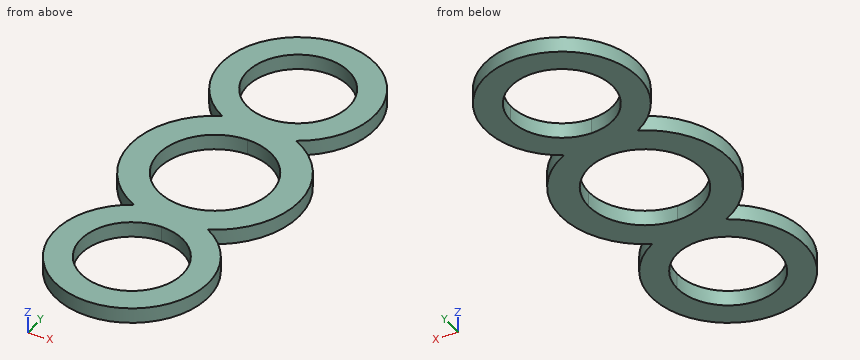
from build123d import *

# Parameters (mm, degrees)
F1_DEPTH = 3


with BuildPart() as f1:
    # F0 (on Top) → F1 (new body)
    with BuildSketch(Plane.XY):
        with BuildLine():
            ThreePointArc((7.205074, 14.84375), (0, 43), (-7.205074, 14.84375))
            ThreePointArc((-7.205074, 14.84375), (-16.5, 0), (-7.205074, -14.84375))
            ThreePointArc((-7.205074, -14.84375), (0, -43), (7.205074, -14.84375))
            ThreePointArc((7.205074, -14.84375), (16.5, 0), (7.205074, 14.84375))
        make_face()
        with BuildLine():
            ThreePointArc((9.95, -28), (-7.035712, -35.035712), (0, -18.05))
            ThreePointArc((0, -18.05), (7.035712, -20.964288), (9.95, -28))
        make_face(mode=Mode.SUBTRACT)
        with BuildLine():
            ThreePointArc((0, 11), (7.778175, 7.778175), (11, 0))
            ThreePointArc((11, 0), (7.778175, -7.778175), (0, -11))
            ThreePointArc((0, -11), (-11, 0), (0, 11))
        make_face(mode=Mode.SUBTRACT)
        with BuildLine():
            ThreePointArc((9.95, 28), (7.035712, 20.964288), (0, 18.05))
            ThreePointArc((0, 18.05), (-7.035712, 35.035712), (9.95, 28))
        make_face(mode=Mode.SUBTRACT)
    extrude(amount=F1_DEPTH)


solid = f1.part
Geometry check sheet. Reference: the model listing, model coordinates, mm. Round coordinates to 2 decimals unless told otherwise and drop trailing zeros. Write each loop counter-clockwise with the first axis right and the second up, starting at its lowest first coordinate (ties: lowest second). Pieces come first, ordered by that corner, then holes.
Item 1: Section check A-A (z = 1.4). Record the boundary of the cut face in (x, y).
Determined:
outline: (-7.21, -14.84) arc R15 ccw (long way) to (7.21, -14.84) arc R16.5 ccw to (7.21, 14.84) arc R15 ccw (long way) to (-7.21, 14.84) arc R16.5 ccw to start; hole (0, -18.05) arc R9.95 ccw (long way) to (9.95, -28) arc R9.95 ccw to start; hole (0, -11) arc R11 ccw to (11, 0) arc R11 ccw to (0, 11) arc R11 ccw to start; hole (0, 18.05) arc R9.95 ccw to (9.95, 28) arc R9.95 ccw (long way) to start
Item 2: Go/stop test with flat-tipped pins: pin 1 Ø1.5 at (x, z) = (-7, 0.5) entering from +Y; pin 2 Ø18 at (x, y) = (0, -28) entering from +Z. Record where each tip stops, or that it passes through.
Determined:
pin 1: stops at y = 41.64
pin 2: passes through
Item 3: Section check C-C (y = 22.5). Record the boundary of the cut face in (x, z).
Determined:
outline: (-13.96, 0) - (-8.29, 0) - (-8.29, 3) - (-13.96, 3) - close; (8.29, 0) - (13.96, 0) - (13.96, 3) - (8.29, 3) - close
Item 4: Material ranges on line 1 along X through (y, z) = (28, 1.7); line 2 along Y through (x, z) = (6.5, 2.6); line 3 along Y through (x, z) = (13, 0.9), recorded low to high.
Determined:
line 1: x = -15 to -9.95, 9.95 to 15
line 2: y = -41.52 to -35.53, -20.47 to -8.87, 8.87 to 20.47, 35.53 to 41.52
line 3: y = -35.48 to -20.52, -10.16 to 10.16, 20.52 to 35.48
Item 5: Section check D-D (y = 34.5). Record the boundary of the cut face in (x, z), plus the area to 3 significant figures.
Determined:
outline: (-13.52, 0) - (-7.53, 0) - (-7.53, 3) - (-13.52, 3) - close; (7.53, 0) - (13.52, 0) - (13.52, 3) - (7.53, 3) - close
area: 35.9 mm2
Item 6: Section check B-B (x = 13.5). Record the boundary of the cut face in (y, z).
Determined:
outline: (-34.54, 0) - (-21.46, 0) - (-21.46, 3) - (-34.54, 3) - close; (-9.49, 0) - (9.49, 0) - (9.49, 3) - (-9.49, 3) - close; (21.46, 0) - (34.54, 0) - (34.54, 3) - (21.46, 3) - close
